Here's how the part is built. I have some questions about the finished solid (model axes, mm). Face numbers are marked on the shaded views. A direction names the side the tool comes from. Give positions to 0.01 mm unless a question says otherwise; leave off trailing zeros. Loops run counter-clockwise (first coordinate to the right, second up) from the corner with the lowest first, then second, coordinate; pieces in that order, holes last. Notation, with made-up numbers: (-13, 25.5) - (46, 25.5) arc R16 cw to (46, 47.5) - close; hole circle Ø4 at (9.25, 75). An arc over 180 degrees is marked (long way). Return JSON: item names as keys, results as strings. Group by question number.
(1) If we section it at C-C (y = -1.25): State how many separate pieces and enclosed holes the cut face has, then the cut area to 3 significant figures.
(2) If we section it at B-B (z = 0): Please give me the cut outline in (x, y).
(3) If we section it at A-A (x = 0): Please give me the cut outline in (y, z).
(4) If we section it at D-D (x = -17): Please give me the cut outline in (y, z), then the cut area to 3 significant figures.
(5) For P1, Ø3, axis at y = -3, z = 17.5, coming from the -X side; P2, Ø4, axis at x = 0.5, y = -6, coming from the +Z side; P3, Ø6, axis at x = -16, z = 0, coming from the +Y side; P4, Ø4.5, axis at x = 3.5, z = 0, coming from the +Y side, each with a flat end and sliding along its axis, tell me the tip position at first contact or that it passes through.
(6) On a 3-axis mill with a long thin cutter (end or side, diameter ignored), from which of +Z, -Z, +X, -X, +Y, -Y can I reach the whole of each face in a straight line? I mean the marked faces 1 and 2. Say none if no direction works.
(7) I need wall thicknesses on probe 1 along Z at (x, y) = (-12, -6.75); probe 2 along Z at (x, y) = (-13, -7.75); probe 3 along X at (y, z) = (-3.75, 2). Which ranges of each line are inside material? Lowest first, please. Write a range as [from, to].
(8) If we mould it in two halves opening along X, with no side actions, what happens to the marked faces 3, 4, 5 and 6? For each: released by +X, released by -X, zero draft, split by the parting line, or undercut.
```python
from build123d import *

# Parameters (mm, degrees)
F0_R     = 22.5
F0_R_2   = 1.5
F1_DEPTH = 10
F2_R     = 7.5
F3_DEPTH = 7
F4_R     = 2.5
F5_DEPTH = 25


with BuildPart() as f1:
    # F0 (on Front) → F1 (new body)
    with BuildSketch(Plane.XZ):
        Circle(F0_R)
        with Locations((-13, -7.5)):
            Circle(F0_R_2, mode=Mode.SUBTRACT)
        with Locations((-7.071068, -7.071068)):
            Circle(F0_R_2, mode=Mode.SUBTRACT)
        with Locations((7.071068, -7.071068)):
            Circle(F0_R_2, mode=Mode.SUBTRACT)
        with Locations((-13, 7.5)):
            Circle(F0_R_2, mode=Mode.SUBTRACT)
        with Locations((-7.071068, 7.071068)):
            Circle(F0_R_2, mode=Mode.SUBTRACT)
        with Locations((0, 10)):
            Circle(F0_R_2, mode=Mode.SUBTRACT)
        with Locations((7.071068, 7.071068)):
            Circle(F0_R_2, mode=Mode.SUBTRACT)
    extrude(amount=F1_DEPTH)

    # F2 (on face) → F3 (cut)
    with BuildSketch(Plane(origin=(0, 0, 0), x_dir=(-1, 0, 0), z_dir=(0, 1, 0))):
        Circle(F2_R)
    extrude(amount=-F3_DEPTH, mode=Mode.SUBTRACT)

    # F4 (on face) → F5 (cut)
    with BuildSketch(Plane.XZ.offset(10)):
        with Locations((0, 16)):
            Circle(F4_R)
        with Locations((16, 0)):
            Circle(F4_R)
        with Locations((0, -16)):
            Circle(F4_R)
        with Locations((-16, 0)):
            Circle(F4_R)
    extrude(amount=-F5_DEPTH, mode=Mode.SUBTRACT)


solid = f1.part
```
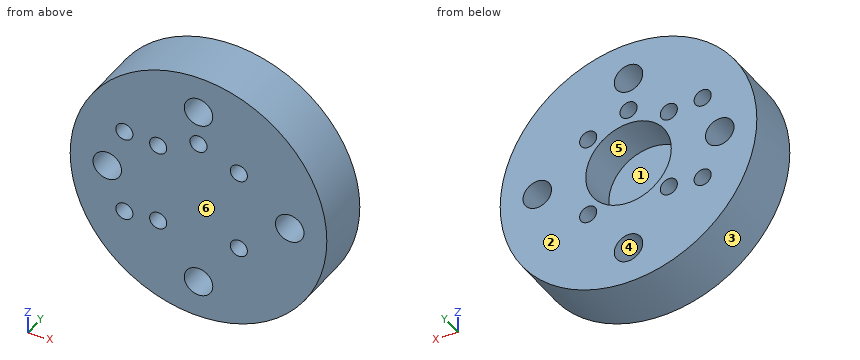
Values:
{
 "1": {"separate pieces": "1", "enclosed holes": "12", "area": "1,290 mm2"},
 "2": {"outline": "(-22.5, -10) - (-18.5, -10) - (-18.5, 0) - (-22.5, 0) - close; (-13.5, -10) - (13.5, -10) - (13.5, 0) - (7.5, 0) - (7.5, -7) - (-7.5, -7) - (-7.5, 0) - (-13.5, 0) - close; (18.5, -10) - (22.5, -10) - (22.5, 0) - (18.5, 0) - close"},
 "3": {"outline": "(-10, -22.5) - (0, -22.5) - (0, -18.5) - (-10, -18.5) - close; (-10, -13.5) - (0, -13.5) - (0, -7.5) - (-7, -7.5) - (-7, 7.5) - (0, 7.5) - (0, 8.5) - (-10, 8.5) - close; (-10, 11.5) - (0, 11.5) - (0, 13.5) - (-10, 13.5) - close; (-10, 18.5) - (0, 18.5) - (0, 22.5) - (-10, 22.5) - close"},
 "4": {"outline": "(-10, -14.74) - (0, -14.74) - (0, -2.29) - (-10, -2.29) - close; (-10, 2.29) - (0, 2.29) - (0, 14.74) - (-10, 14.74) - close", "area": "249 mm2"},
 "5": {"P1": "x = -15.82", "P2": "z = 22.5", "P3": "y = 0", "P4": "y = -7"},
 "6": {"face 1": "+Y", "face 2": "+Z, -Z, +X, -X, +Y"},
 "7": {"probe 1": "[-19.03, -8.62], [-6.38, 6.38], [8.62, 19.03]", "probe 2": "[-18.36, -9], [-6, 6], [9, 18.36]", "probe 3": "[-22.41, -17.5], [-14.5, -7.23], [7.23, 14.5], [17.5, 22.41]"},
 "8": {"face 3": "split by the parting line", "face 4": "undercut", "face 5": "undercut", "face 6": "zero draft"}
}
